```python
from build123d import *

# Parameters (mm, degrees)
SKETCH1_R           = 14.9606
BOSS_EXTRUDE1_DEPTH = 4.7625
SKETCH2_R           = 2.5527
CUT_EXTRUDE1_DEPTH  = 6.35
SKETCH3_R           = 1.5875
CUT_EXTRUDE2_DEPTH  = 10
SKETCH5_R           = 15.875
SKETCH5_R_2         = 14.9606
BOSS_EXTRUDE2_DEPTH = 1.5875
CUT_EXTRUDE3_DEPTH  = 2.54


with BuildPart() as part:
    # Sketch1 → Boss-Extrude1 (new body)
    with BuildSketch(Plane(origin=(234.278878836, -18.689027227, 0), x_dir=(0, 0, -1), z_dir=(0.9968332748770866, -0.0795199477981641, 0))):
        with Locations(Location((-43.174261814, 8.550344032, 0), (0, 0, 90))):
            Circle(SKETCH1_R)
    extrude(amount=-BOSS_EXTRUDE1_DEPTH)

    # Sketch2 → Cut-Extrude1 (cut)
    with BuildSketch(Plane(origin=(234.278878836, -18.689027227, 0), x_dir=(0, 0, -1), z_dir=(0.9968332748770866, -0.07951994779816411, 0))):
        with Locations(Location((-43.174261814, 8.550344032, 0), (0, 0, 90))):
            Circle(SKETCH2_R)
    extrude(amount=-CUT_EXTRUDE1_DEPTH, mode=Mode.SUBTRACT)

    # Sketch3 → Cut-Extrude2 (cut)
    with BuildSketch(Plane(origin=(229.531460364, -18.310313476, 0), x_dir=(0, 0, 1), z_dir=(-0.9968332748770866, 0.07951994779816411, 0))):
        with Locations(Location((30.474261814, 8.550344032, 0), (0, 0, 270))):
            Circle(SKETCH3_R)
        with Locations(Location((43.174261814, 21.250344032, 0), (0, 0, 270))):
            Circle(SKETCH3_R)
        with Locations(Location((52.154517935, 17.530600153, 0), (0, 0, 270))):
            Circle(SKETCH3_R)
        with Locations(Location((55.874261814, 8.550344032, 0), (0, 0, 270))):
            Circle(SKETCH3_R)
        with Locations(Location((52.154517935, -0.429912089, 0), (0, 0, 270))):
            Circle(SKETCH3_R)
        with Locations(Location((43.174261814, -4.149655968, 0), (0, 0, 270))):
            Circle(SKETCH3_R)
        with Locations(Location((34.194005693, -0.429912089, 0), (0, 0, 270))):
            Circle(SKETCH3_R)
        with Locations(Location((34.194005693, 17.530600153, 0), (0, 0, 270))):
            Circle(SKETCH3_R)
    extrude(amount=-CUT_EXTRUDE2_DEPTH, mode=Mode.SUBTRACT)

    # Sketch5 → Boss-Extrude2 (add)
    with BuildSketch(Plane(origin=(234.278878836, -18.689027227, 0), x_dir=(0, 0, 1), z_dir=(-0.9968332748770866, 0.07951994779816411, 0))):
        with Locations(Location((43.174261814, 8.550344032, 0), (0, 0, 270))):
            Circle(SKETCH5_R)
        with Locations(Location((43.174261814, 8.550344032, 0), (0, 0, 90))):
            Circle(SKETCH5_R_2, mode=Mode.SUBTRACT)
    extrude(amount=BOSS_EXTRUDE2_DEPTH)

    # Sketch6 → Cut-Extrude3 (cut)
    with BuildSketch(Plane(origin=(234.278878836, -18.689027227, 0), x_dir=(0, 0, -1), z_dir=(0.9968332748770866, -0.07951994779816411, 0))):
        Polygon((-133.921695756, 23.510944032), (-48.484259238, 23.510944032), (-37.864264391, 23.510944032), (47.573172128, 23.510944032), (47.573172128, 194.385817069), (-133.921695756, 194.385817069), align=None)
    extrude(amount=-CUT_EXTRUDE3_DEPTH, mode=Mode.SUBTRACT)


solid = part.part
```
Here's how the part is built. I have some questions about the finished solid (model axes, mm). Give positions to 0.01 mm unless a question says otherwise; leave off trailing zeros. Order: outer loops, then holes, each group sorted by start corner. A loop starts at its lowest first (then second) coordinate and runs counter-clockwise, first axis right, second up. Notation, with made-up numbers: (8, 2.25) - (28, 2.25) arc R16 cw to (28, 32.25) - close; hole circle Ø1 at (44.25, 68.5). An arc over 180 degrees is marked (long way). Answer as a JSON object with one key per item and string values. Group by question number.
Item 1: If we section it at B-B on z = 46.5: Please give me the cut outline in (x, y).
Item 2: If we section it at A-A on z = 41: Please give me the cut outline in (x, y), and give its area (3 significant figures).
Item 3: For P1, Ø2, axis at x = 230.5, z = 50, coming from the -Y side; P2, Ø4, axis at y = -14, z = 54, coming from the +X side; P3, Ø2, axis at y = 1.5, z = 40.5, coming from the +X side, each with a flat end and sliding along its axis, tell me the tip position at first contact or that it passes through.
Item 4: If we section it at C-C on y = 0: Give the number of separate pieces and of enclosed holes in the cut face, and give its area (3 significant figures).
Item 5: Please list where these lines run through material, in increasing order: probe 1 along Z at (x, y) = (234.25, -10); probe 2 along Z at (x, y) = (234.5, 0); probe 3 along Z at (x, y) = (233.25, 0).
Item 6: If we section it at D-D on z = 31.5: Please give me the cut outline in (x, y).
Item 7: If we mould it in two halves opening along Y, with no side actions, what happens to faces 1 (the cylindrical face through (232.592, -10.31, 45.705)), 2 (the flat face through (232.256, -24.085, 37.369)), 3 (the cylindrical face through (232.917, -25.916, 42.552)), 4 (the flat face through (235.37, 4.81, 43.25))? For each: pulls with the +Y half, pulls with the -Y half, needs draft (parallel to the pull), parting line crosses it, or undercut.
Result set:
{
 "1": {"outline": "(229.05, -24.33) - (232.22, -24.58) - (232.14, -25.51) - (233.72, -25.64) - (236.15, 4.75) - (234.57, 4.87) - (234.54, 4.5) - (231.37, 4.75) - close"},
 "2": {"outline": "(229.03, -24.54) - (232.2, -24.79) - (232.13, -25.72) - (233.71, -25.84) - (234.85, -11.5) - (230.11, -11.12) - close; (230.32, -8.45) - (235.07, -8.83) - (236.15, 4.75) - (234.57, 4.87) - (234.55, 4.72) - (231.39, 4.97) - close", "area": "130 mm²"},
 "3": {"P1": "y = -23.64", "P2": "x = 234.81", "P3": "x = 235.97"},
 "4": {"separate pieces": "3", "enclosed holes": "0", "area": "87.2 mm²"},
 "5": {"probe 1": "27.3 to 28.89, 32.06 to 40.62, 45.72 to 54.29, 57.46 to 59.05", "probe 2": "30.92 to 33.07, 35.32 to 51.03, 53.28 to 55.42", "probe 3": "32.04 to 32.98, 35.41 to 50.94, 53.37 to 54.3"},
 "6": {"outline": "(229.47, -19.11) - (232.63, -19.37) - (232.52, -20.76) - (234.1, -20.89) - (234.86, -11.37) - (230.12, -10.99) - close; (230.31, -8.58) - (235.06, -8.96) - (235.81, 0.56) - (234.23, 0.68) - (234.12, -0.71) - (230.96, -0.46) - close"},
 "7": {"face 1": "undercut", "face 2": "undercut", "face 3": "parting line crosses it", "face 4": "pulls with the +Y half"}
}
